Geometry check sheet. Reference: the model listing, model coordinates, mm. A direction names the side the tool comes from. Round coordinates to 2 decimals unless told otherwise and drop trailing zeros. Write each loop counter-clockwise with the first axis right and the second up, starting at its lowest first coordinate (ties: lowest second). Pieces come first, ordered by that corner, then holes. Notation, with made-up numbers: M -23,-13.75 L -15,-13.75 A10 cw -15,4.25 Z; hole C -32.75,48 d1. An arc over 180 degrees is marked long. Put each result on its own line as item: value. Start each with the question number.
(1) Section check D-D on x = 153.5. Record the cut outline in (y, z).
(2) Section check B-B on z = 10. Record the cut outline in (x, y), then the cut area to 3 significant figures.
(3) Gauge pin test, flat ends, axial feed: pin 1 (8 mm diameter, centred on x = 150, z = 7.5, fed in from +Y); pin 2 (2 mm diameter, centred on y = -0.5, z = 34.5, fed in from -X); pin 3 (2 mm diameter, centred on y = -7.5, z = -24, fed in from -X). Record the tip position at first contact, or that the pin passes through.
(4) Tool access check on faces 4 (the flat face through (207.962, -6, 43)), 5 (the cylindrical face through (-193.974, 3.131, -35.619)), 6 (the flat face through (-15, -12.7, -15)), 7 (the flat face through (207, 0, -4)). Record the directions out of +Z, -Z, +X, -X, +Y, -Y that give a thin tool (end or side, any length) a straight path to the whole face; none if there is none.
(5) Section check A-A on x = 79. Record the cut outline in (y, z).
(6) Section check C-C on y = -7.5. Record the cut outline in (x, z).
(7) Mould release check, pull along X, two halves, no side actions. Record for faces 1 (the flat face through (122.238, -6, 24)), 2 (the flat face through (137, -6, 55.562)), 3 (the flat face through (-227.012, -6, 10)): pulls with the +X half, pulls with the -X half, needs draft (parallel to the pull), parting line crosses it, or undercut.
(8) Material ranges on probe 1 along X at (y, z) = (-3.25, 22); probe 2 along Z at (x, y) = (-95, -9.25); probe 3 along Z at (x, y) = (-137, 5), recorded low to high.
from build123d import *

# Parameters (mm, degrees)
F0_R          = 8.8265
F1_DEPTH      = 12.7
F3_DEPTH      = 6.35
F3_DEPTH_BACK = 19.05


with BuildPart() as f1:
    # F0 (on Front) → F1 (new body)
    with BuildSketch(Plane.XZ):
        with BuildLine():
            Line((227.0125, 30.1625), (220.6625, 55.5625))
            Line((220.6625, 55.5625), (207.9625, 55.5625))
            Line((207.9625, 55.5625), (207.9625, 30.1625))
            ThreePointArc((207.9625, 30.1625), (198.66314, 7.71186), (176.2125, -1.5875))
            ThreePointArc((176.2125, -1.5875), (153.76186, 7.71186), (144.4625, 30.1625))
            Line((144.4625, 30.1625), (144.4625, 55.5625))
            Line((144.4625, 55.5625), (128.5875, 55.5625))
            Line((128.5875, 55.5625), (122.2375, 30.1625))
            Line((122.2375, 30.1625), (122.2375, 17.4625))
            ThreePointArc((122.2375, 17.4625), (118.517756, 8.482244), (109.5375, 4.7625))
            Line((109.5375, 4.7625), (-176.2125, 4.7625))
            ThreePointArc((-176.2125, 4.7625), (-194.173012, 12.201988), (-201.6125, 30.1625))
            Line((-201.6125, 30.1625), (-227.0125, 30.1625))
            Line((-227.0125, 30.1625), (-227.0125, -11.1125))
            ThreePointArc((-227.0125, -11.1125), (-213.993396, -42.543396), (-182.5625, -55.5625))
            Line((-182.5625, -55.5625), (214.3125, -55.5625))
            ThreePointArc((214.3125, -55.5625), (223.292756, -51.842756), (227.0125, -42.8625))
            Line((227.0125, -42.8625), (227.0125, 30.1625))
        make_face()
        with Locations((-138.1125, -24.511)):
            Circle(F0_R, mode=Mode.SUBTRACT)
    extrude(amount=F1_DEPTH)

    # F2 (on face) → F3 (join, two sides)
    with BuildSketch(Plane.XZ.offset(12.7)) as f3_sk:
        with BuildLine():
            Line((-201.6125, -17.4625), (-201.6125, 30.1625))
            Line((-201.6125, 30.1625), (-227.0125, 30.1625))
            Line((-227.0125, 30.1625), (-227.0125, -11.1125))
            ThreePointArc((-227.0125, -11.1125), (-213.993396, -42.543396), (-182.5625, -55.5625))
            Line((-182.5625, -55.5625), (214.3125, -55.5625))
            ThreePointArc((214.3125, -55.5625), (223.292756, -51.842756), (227.0125, -42.8625))
            Line((227.0125, -42.8625), (185.7375, -42.8625))
            Line((185.7375, -42.8625), (180.935652, -5.739069))
            ThreePointArc((180.935652, -5.739069), (176.2125, -1.5875), (171.489348, -5.739069))
            Line((171.489348, -5.739069), (166.6875, -42.8625))
            Line((166.6875, -42.8625), (-176.2125, -42.8625))
            ThreePointArc((-176.2125, -42.8625), (-194.173012, -35.423012), (-201.6125, -17.4625))
        make_face()
    extrude(amount=F3_DEPTH)
    extrude(f3_sk.sketch, amount=-F3_DEPTH_BACK)


solid = f1.part
Answers follow:
1. outline: M -19.05,-55.56 L 6.35,-55.56 L 6.35,-42.86 L 0,-42.86 L 0,7.98 L -12.7,7.98 L -12.7,-42.86 L -19.05,-42.86 Z
2. outline: M -227.01,-19.05 L -201.61,-19.05 L -201.61,-12.7 L -191.66,-12.7 L -191.66,0 L -201.61,0 L -201.61,6.35 L -227.01,6.35 Z; M 119.81,-12.7 L 151.69,-12.7 L 151.69,0 L 119.81,0 Z; M 200.74,-12.7 L 227.01,-12.7 L 227.01,0 L 200.74,0 Z
2. area: 1,510 mm^2
3. pin 1: stops at y = 0
3. pin 2: stops at x = 123.07
3. pin 3: stops at x = -225.39
4. face 4: +Z, +Y, -Y
4. face 5: +Z, +Y
4. face 6: +Z, -Y
4. face 7: +Z, +X, +Y
5. outline: M -19.05,-55.56 L 6.35,-55.56 L 6.35,-42.86 L 0,-42.86 L 0,4.76 L -12.7,4.76 L -12.7,-42.86 L -19.05,-42.86 Z
6. outline: M -227.01,-11.11 A44.45 ccw -182.56,-55.56 L 214.31,-55.56 A12.7 ccw 227.01,-42.86 L 227.01,30.16 L 220.66,55.56 L 207.96,55.56 L 207.96,30.16 A31.75 cw 176.21,-1.59 A31.75 cw 144.46,30.16 L 144.46,55.56 L 128.59,55.56 L 122.24,30.16 L 122.24,17.46 A12.7 cw 109.54,4.76 L -176.21,4.76 A25.4 cw -201.61,30.16 L -227.01,30.16 Z; hole C -138.11,-24.51 d17.65
7. face 1: undercut
7. face 2: needs draft
7. face 3: pulls with the -X half
8. probe 1: x = -227.01 to -200.27, 122.24 to 145.53, 206.9 to 227.01
8. probe 2: z = -55.56 to 4.76
8. probe 3: z = -55.56 to -42.86
